Check sheet for the modelled part. Datum: model origin and axes. Units: mm. Round coordinates to 2 decimals unless told otherwise and drop trailing zeros. Loops run counter-clockwise (first coordinate to the right, second up) from the corner with the lowest first, then second, coordinate; pieces in that order, holes last. Notation, with made-up numbers: (87.5, -7.75) -> (146.5, -7.75) arc R13 cw to (146.5, 14.25) -> close; hole circle Ø7 at (36.5, 83). An arc over 180 degrees is marked (long way). Use one line per item in the form item = value. Start each with the question number.
(1) Sectioned sample at C-C (x = -3). Record the cut outline in (y, z), and give its area (3 significant figures).
(2) Material ranges on probe 1 along Z at (x, y) = (-1.75, 13.25); probe 2 along Y at (x, z) = (0.5, 7.75); probe 3 along Y at (x, z) = (-1, 4), recorded low to high. Write a range as [from, to].
(3) Sectioned sample at D-D (z = 3.5). Record the cut outline in (x, y), and give its area (3 significant figures).
(4) Sectioned sample at B-B (z = 6). Record the cut outline in (x, y), and give its area (3 significant figures).
(5) Go/stop test with flat-tipped pins: pin 1 (5 mm diameter, centred on y = 7, z = 9, fed in from -X); pin 2 (2 mm diameter, centred on x = 6, z = 7, fed in from -Y). Record where each tip stops, or that it passes through.
(6) Sectioned sample at A-A (x = 1). Record the cut outline in (y, z).
Autodesk Inventor part; units mm, degrees
ref_plane "YZ Plane" through (0, 0, 0) normal (1, 0, 0) x (0, 1, 0)
ref_plane "XZ Plane" through (0, 0, 0) normal (0, 1, 0) x (-1, 0, 0)
ref_plane "XY Plane" through (0, 0, 0) normal (0, 0, 1) x (1, 0, 0)
sketch "Sketch1" plane through (0, 0, 0) normal (0, 0, 1) x (1, 0, 0)
  line L0 (-6.32, 0) -> (-9.14, 15.933)
  line L1 (-9.14, 15.933) -> (9.14, 15.933)
  line L2 (9.14, 15.933) -> (6.32, 0)
  line L3 (6.32, 0) -> (-6.32, 0)
  point P0 (0, 0)
  point P1 (0, 15.933)
  point P2 (0, 0)
  dimension "d0" = 2.82
  dimension "d1" = 15.933
  dimension "d2" = 12.64
extrude "Extrusion1" add sketch "Sketch1" along normal blind 12.7
fillet "Fillet1" radius 2 4 edges at (0, 0, 0) (6.32, 0, 6.35) (0, 0, 12.7) (-6.32, 0, 6.35)
fillet "Fillet2" radius 1 12 edges at (7.907, 8.9665, 12.7) (5.928, 0.4675, 11.9851) (6.643, 1.825, 12.6923) (5.928, 0.4675, 0.7149) (7.907, 8.9665, 0) (6.643, 1.825, 0.0077) (-6.643, 1.825, 0.0077) (-7.907, 8.9665, 0) (-5.928, 0.4675, 0.7149) (-5.928, 0.4675, 11.9851) (-7.907, 8.9665, 12.7) (-6.643, 1.825, 12.6923)
sketch "Sketch2" plane through (-8.1245, 15.933, 0) normal (0, 1, 0) x (1, 0, 0)
  arc A0 (8.1245, -2.35) -> (8.1245, -10.35) centre (8.1245, -6.35) ccw
  line L0 (16.2489, 0) -> (0, 0)
  line L1 (8.1245, -10.35) -> (8.1245, -2.35)
  line L2 (-1.0155, -1) -> (-1.0155, -11.7)
  point P0 (8.1245, 0)
  point P1 (8.1245, 0)
  point P2 (-1.0155, -6.35)
  dimension "d7" = 4
revolve "Revolution1" cut sketch "Sketch2" angle 135 about axis through (0, 15.933, 10.35) along (0, 0, 1)
properties part number "OwnSpectr_TubeHolder_D_3DPrint"
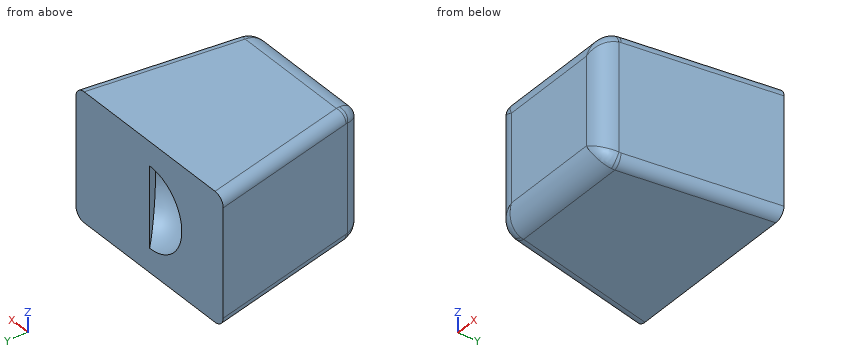
Checks:
q1.outline = (0, 2) arc R2 ccw to (2, 0) -> (15.93, 0) -> (15.93, 3.7) arc R2.65 cw to (15.93, 9) -> (15.93, 12.7) -> (2, 12.7) arc R2 ccw to (0, 10.7) -> close
q1.area = 190 mm2
q2.probe_1 = [0, 3.95], [8.75, 12.7]
q2.probe_2 = [0, 12.22], [15.43, 15.93]
q2.probe_3 = [0, 12.85]
q3.outline = (-9.14, 15.93) -> (-6.61, 1.65) arc R2 ccw to (-4.64, 0) -> (4.64, 0) arc R2 ccw to (6.61, 1.65) -> (9.14, 15.93) -> (0, 15.93) -> (1.98, 13.95) arc R2.81 cw to (-2.81, 15.93) -> close
q3.area = 236 mm2
q4.outline = (-9.14, 15.93) -> (-6.61, 1.65) arc R2 ccw to (-4.64, 0) -> (4.64, 0) arc R2 ccw to (6.61, 1.65) -> (9.14, 15.93) -> (0, 15.93) -> (2.82, 13.12) arc R3.98 cw to (-3.98, 15.93) -> close
q4.area = 226 mm2
q5.pin_1 = -8
q5.pin_2 = 0.03
q6.outline = (0, 2) arc R2 ccw to (2, 0) -> (15.93, 0) -> (15.93, 12.7) -> (2, 12.7) arc R2 ccw to (0, 10.7) -> close; hole (14.93, 2.61) -> (14.93, 10.09) arc R3.87 ccw to start
